Autodesk Inventor part; units mm, degrees
ref_plane "YZ Plane" through (0, 0, 0) normal (1, 0, 0) x (0, 1, 0)
ref_plane "XZ Plane" through (0, 0, 0) normal (0, 1, 0) x (-1, 0, 0)
ref_plane "XY Plane" through (0, 0, 0) normal (0, 0, 1) x (1, 0, 0)
sketch "スケッチ1" plane through (0, 0, 0) normal (0, 1, 0) x (-1, 0, 0)
  line L0 (-16, -13) -> (16, -13)
  line L1 (16, -13) -> (16, 13)
  line L2 (16, 13) -> (-16, 13)
  line L3 (-16, 13) -> (-16, -13)
  line L4 (-16, -13) -> (16, 13) construction
  line L5 (16, -13) -> (-16, 13) construction
  line L6 (-14, -8) -> (14, -8) construction
  line L7 (14, -8) -> (14, 8)
  line L8 (14, 8) -> (-14, 8) construction
  line L9 (-14, 8) -> (-14, -8)
  line L10 (-14, -8) -> (14, 8) construction
  line L11 (14, -8) -> (-14, 8) construction
  circle A0 centre (14, -8) radius 0.8
  circle A1 centre (14, 8) radius 0.8
  circle A2 centre (-14, -8) radius 0.8
  circle A3 centre (-14, 8) radius 0.8
  point P0 (0, 0)
  dimension "d0" = 32
  dimension "d1" = 26
  dimension "d2" = 28
  dimension "d3" = 16
  dimension "d4" = 1.6
  dimension "d5" = 1.6
  dimension "d6" = 1.6
  dimension "d7" = 1.6
extrude "押し出し1" add sketch "スケッチ1" along normal blind 2
sketch "スケッチ2" plane through (0, 2, 0) normal (0, 1, 0) x (1, 0, 0)
  circle A0 centre (0, 0) radius 6 construction
  circle A1 centre (0, 0) radius 10
  circle A2 centre (-6, 0) radius 0.8
  circle A3 centre (-4.2426, -4.2426) radius 0.8
  circle A4 centre (0, -6) radius 0.8
  circle A5 centre (4.2426, -4.2426) radius 0.8
  circle A6 centre (6, 0) radius 0.8
  circle A7 centre (4.2426, 4.2426) radius 0.8
  circle A8 centre (0, 6) radius 0.8
  circle A9 centre (-4.2426, 4.2426) radius 0.8
  dimension "d10" = 12
  dimension "d11" = 20
  dimension "d12" = 1.6
  dimension "d15" = 360
extrude "押し出し2" add sketch "スケッチ2" along normal blind 4
fillet "フィレット1" radius 4 1 edges at (-10, 2, 0)
fillet "フィレット2" radius 3 4 edges at (16, 1, 13) (16, 1, -13) (-16, 1, 13) (-16, 1, -13)
properties part number "neck"
Geometry check sheet. Reference: the model listing, model coordinates, mm. A direction names the side the tool comes from. Give positions to 0.01 mm unless a question says otherwise; leave off trailing zeros. Order: outer loops, then holes, each group sorted by start corner. A loop starts at its lowest first (then second) coordinate and runs counter-clockwise, first axis right, second up.
1. Thickness scan on L1, parallel to X at y = 0.95, z = 8; L2, parallel to Z at x = 0, y = 3.75; L3, parallel to X at y = 4, z = 0. Record the ranges inside material, lowest first.
2. Section check B-B, the plane y = 3.75. Give the number of separate pieces and of enclosed holes in the cut face, and give its area (3 significant figures).
3. Section check A-A, the plane x = 0. Enter the section's corners in (y, z).
4. Release check for a two-part mould opening along Z. For faces 1 (the face through (14.59, 0.99, -8.54)), 2 (the face through (-15, 2, 0)), 3 (the face through (-15.14, 1.01, 12.1)) record: pulls with the +Z half, pulls with the -Z half, needs draft (parallel to the pull), parting line crosses it, or undercut.
5. Gauge pin test, flat ends, axial feed: pin 1 Ø1.8 at (x, z) = (-14, -8) entering from +Y; pin 2 Ø3 at (x, z) = (-11.5, 3.5) entering from +Y; pin 3 Ø1.5 at (x, y) = (-0.5, 5) entering from +Z. Record the tip position at first contact, or that the pin passes through.
6. Access from +Z, -Z, +X, -X, +Y, -Y to the whole of each face (thin tool, end or side, straight path). Record for faces 4 (the face through (-4, 2, 4)), 5 (the face through (14.59, 0.99, 7.46)), 6 (the face through (14.3, 2, 0.2)).
Values follow:
1. L1: x = -16 to -14.8, -13.2 to 13.2, 14.8 to 16
1. L2: z = -10.69 to -6.8, -5.2 to 5.2, 6.8 to 10.69
1. L3: x = -10.54 to -6.8, -5.2 to 5.2, 6.8 to 10.54
2. separate pieces: 1
2. enclosed holes: 8
2. area: 343 mm2
3. outline: (0, -13) - (2.13, -13) arc R4 cw to (6, -10) - (6, -6.8) - (2, -6.8) - (2, -5.2) - (6, -5.2) - (6, 5.2) - (2, 5.2) - (2, 6.8) - (6, 6.8) - (6, 10) arc R4 cw to (2.13, 13) - (0, 13) - close
4. face 1: undercut
4. face 2: needs draft
4. face 3: pulls with the +Z half
5. pin 1: stops at y = 2
5. pin 2: stops at y = 4.03
5. pin 3: stops at z = 10.39
6. face 4: +Y
6. face 5: +Y, -Y
6. face 6: +X, +Y
